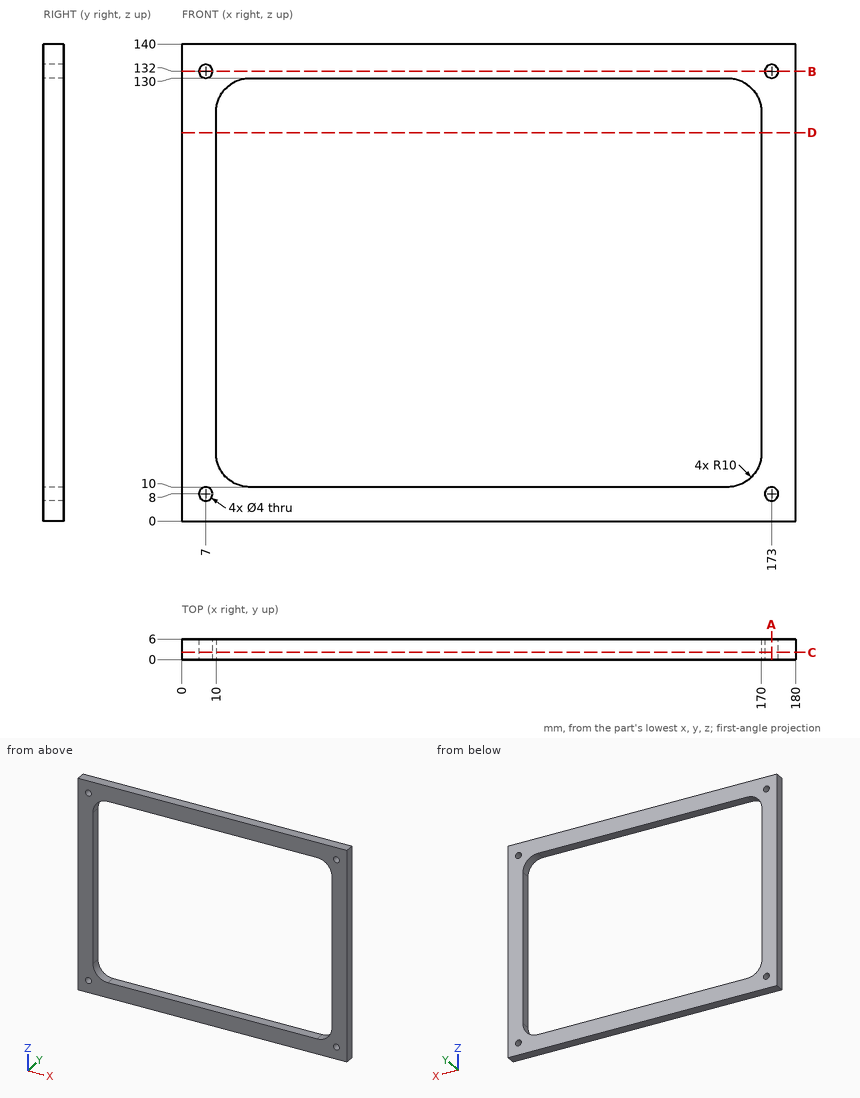
Study the drawing (mm; zero at the part's minimum x, y, z) and answer. Give positions to 0.01 mm unless a question says otherwise; leave off trailing zeros. Loops run counter-clockwise (first coordinate to the right, second up) from the corner with the lowest first, then second, coordinate; pieces in that order, holes last. Notation, with made-up numbers: (75.25, 34) -> (115.25, 34) arc R25 cw to (115.25, 67) -> close; hole circle Ø2 at (11.5, 48). An arc over 180 degrees is marked (long way). Write item = value, one per line. Start each with the question number.
(1) Given pin 1 Ø3 at (x, y) = (111.5, 3) entering from -Z; pin 2 Ø2.5 at (x, z) = (7, 8) entering from -Y, each flat-ended and moving along its own axis, determine where each tip first touches the part or whether it passes through.
(2) Find section C-C on y = 2.1. Give the vertices of the cut face in (x, z).
(3) Find the intervals of material crossed by probe 1 along Z at (x, y) = (7, 3.9); probe 2 along X at (y, z) = (2, 132); probe 3 along X at (y, z) = (3.65, 74.5), in increasing order. Write a range as from..to.
(4) Find section B-B on z = 132. Give the vertices of the cut face in (x, y).
(5) Find section A-A on x = 173. Give the vertices of the cut face in (y, z).
(6) Find section D-D on z = 114. Give the vertices of the cut face in (x, y).
From the geometry:
q1.pin_1 = 0
q1.pin_2 = through
q2.outline = (0, 0) -> (180, 0) -> (180, 140) -> (0, 140) -> close; hole circle Ø4 at (7, 8); hole circle Ø4 at (7, 132); hole (10, 20) arc R10 ccw to (20, 10) -> (160, 10) arc R10 ccw to (170, 20) -> (170, 120) arc R10 ccw to (160, 130) -> (20, 130) arc R10 ccw to (10, 120) -> close; hole circle Ø4 at (173, 8); hole circle Ø4 at (173, 132)
q3.probe_1 = 0..6, 10..130, 134..140
q3.probe_2 = 0..5, 9..171, 175..180
q3.probe_3 = 0..10, 170..180
q4.outline = (0, 0) -> (5, 0) -> (5, 6) -> (0, 6) -> close; (9, 0) -> (171, 0) -> (171, 6) -> (9, 6) -> close; (175, 0) -> (180, 0) -> (180, 6) -> (175, 6) -> close
q5.outline = (0, 0) -> (6, 0) -> (6, 6) -> (0, 6) -> close; (0, 10) -> (6, 10) -> (6, 130) -> (0, 130) -> close; (0, 134) -> (6, 134) -> (6, 140) -> (0, 140) -> close
q6.outline = (0, 0) -> (10, 0) -> (10, 6) -> (0, 6) -> close; (170, 0) -> (180, 0) -> (180, 6) -> (170, 6) -> close
